Could you check a few things on this model? Use its own coordinates, in mm. A direction names the side the tool comes from. Give positions to 0.01 mm unless a question says otherwise; leave off trailing zeros. Order: outer loops, then holes, each group sorted by start corner. A loop starts at its lowest first (then second) coordinate and runs counter-clockwise, first axis right, second up. Notation, with made-up numbers: M 60.5,10.5 L 99.5,10.5 A23 cw 99.5,28.5 Z; hole C 58,-21.5 d7. An arc over 180 degrees is marked long. Answer in a Markdown table with one row per item. Add a question column.
Autodesk Inventor part; units mm, degrees
ref_plane "Work Plane1" through (0, 0, 8) normal (0, 0, 1) x (1, 0, 0)
ref_plane "YZ Plane" through (0, 0, 0) normal (1, 0, 0) x (0, 1, 0)
ref_plane "XZ Plane" through (0, 0, 0) normal (0, 1, 0) x (-1, 0, 0)
sketch "Sketch1" plane through (0, 0, 0) normal (0, 0, 1) x (1, 0, 0)
  line L0 (-17.75, 0) -> (17.75, 0)
  line L1 (17.75, 0) -> (17.75, -85)
  line L2 (17.75, -85) -> (-17.75, -85)
  line L3 (-17.75, -85) -> (-17.75, 0)
  point P0 (0, 0)
  point P1 (0, 0)
  dimension "d0" = 35.5
  dimension "d1" = 85
extrude "Extrusion1" add sketch "Sketch1" along normal blind 11
sketch "Sketch2" plane through (0, 0, 0) normal (1, 0, 0) x (0, 1, 0)
  line L0 (-85, 0) -> (0, 0)
  line L1 (-85, 0) -> (-85, 11)
  line L2 (0, 11) -> (-85, 11)
  line L3 (0, 0) -> (0, 11)
  line L4 (-85, 82.7102) -> (-37.2472, 0)
  line L5 (0, 0) -> (0, 11)
  line L6 (0, 9) -> (-9, 9)
  line L7 (-9, 9) -> (-13.1212, 7.5)
  line L8 (-13.1212, 7.5) -> (-22, 7.5)
  line L9 (-22, 7.5) -> (-24.7475, 6.5)
  line L10 (-24.7475, 6.5) -> (-41, 6.5)
  line L11 (-45.9075, 15) -> (-85, 15)
  line L12 (-85, 15) -> (-85, 11)
  point P0 (-43.5981, 11)
  dimension "d6" = 60
  dimension "d7" = 20
  dimension "d8" = 2
  dimension "d9" = 3.5
  dimension "d10" = 4.5
  dimension "d11" = 6.5
  dimension "d12" = 9
  dimension "d13" = 13.1212
  dimension "d14" = 24.7475
  dimension "d15" = 22
  dimension "d16" = 41
  dimension "d25" = 15
  dimension "d26" = 4
extrude "Extrusion2" add sketch "Sketch2" along normal mid plane 60 contours L1 L2 L4 L0 | L12 L11 L4 L2
extrude "Extrusion4" add sketch "Sketch2" along normal mid plane 43.6 contours L4 L2 L3 L6 L7 L8 L9 L10
sketch "Sketch3" plane through (0, 0, 0) normal (0, 0, 1) x (1, 0, 0)
  line L0 (-13, 13) -> (13, 13)
  line L1 (-17.75, 0) -> (17.75, 0)
  line L2 (-30, -37.2472) -> (-30, -85)
  line L3 (30, -85) -> (30, -37.2472)
  line L4 (30, -85) -> (-30, -85)
  arc A0 (-13, 13) -> (-30, -4) centre (-13, -4) ccw
  arc A1 (30, -4) -> (13, 13) centre (13, -4) ccw
  line L5 (-30, -37.2472) -> (-30, -4)
  line L6 (30, -37.2472) -> (30, -4)
  point P0 (0, 0)
  dimension "d28" = 13
  dimension "d29" = 17
extrude "Extrusion5" add sketch "Sketch3" against normal blind 3
fillet "Fillet1" radius 3 1 edges at (0, -45.9075, 15)
fillet "Fillet2" radius 2 2 edges at (23.875, -37.2472, 0) (-23.875, -37.2472, 0)
sketch "Sketch4" plane through (0, 0, 11) normal (0, 0, 1) x (1, 0, 0)
  line L0 (21.8, -43.5981) -> (-21.8, -43.5981)
  line L1 (21.8, 0) -> (21.8, -43.5981)
  line L2 (21.8, 0) -> (-21.8, 0)
  line L3 (-21.8, -43.5981) -> (-21.8, 0)
  line L4 (-21.8, -43.5981) -> (-21.8, 0)
  line L5 (-21.8, -9) -> (-17.75, -2)
  line L6 (-21.8, -9) -> (-13.7128, -9) construction
  line L7 (-17.75, -2) -> (-17.75, 0)
  line L8 (21.8, 0) -> (-21.8, 0)
  point P0 (0, 0)
  dimension "d34" = 2
extrude "Extrusion6" cut sketch "Sketch4" against normal up to next contours L3 L2 L7 L5
mirror "Mirror1" about plane through (0, 0, 0) normal (1, 0, 0) of "Extrusion6"
sketch "Sketch5" plane through (0, 0, 11) normal (0, 0, 1) x (1, 0, 0)
  line L0 (0.95, 0) -> (-0.95, 0)
  line L1 (-0.95, 0) -> (-0.95, -17)
  line L2 (-0.95, -17) -> (0.95, -17)
  line L3 (0.95, -17) -> (0.95, 0)
  line L4 (8.45, 0) -> (6.55, 0)
  line L5 (6.55, 0) -> (6.55, -17)
  line L6 (6.55, -17) -> (8.45, -17)
  line L7 (8.45, -17) -> (8.45, 0)
  line L8 (-6.55, 0) -> (-8.45, 0)
  line L9 (-8.45, 0) -> (-8.45, -17)
  line L10 (-8.45, -17) -> (-6.55, -17)
  line L11 (-6.55, -17) -> (-6.55, 0)
  line L12 (17.75, 0) -> (-17.75, 0)
  point P0 (0, 0)
  point P1 (7.5, 0)
  point P2 (-7.5, 0)
  point P3 (0, 0)
  dimension "d37" = 7.5
  dimension "d38" = 7.5
  dimension "d39" = 1.9
  dimension "d40" = 17
extrude "Extrusion7" cut sketch "Sketch5" against normal up to surface (14 mm away)
ref_plane "Work Plane1" through (0, 0, 8) normal (0, 0, 1) x (1, 0, 0)
sketch "Sketch8" plane through (-30, -85, 15) normal (0, 0, 1) x (1, 0, 0)
  line L0 (14.5, 54.9) -> (14.5, 44)
  line L1 (14.5, 44) -> (45.5, 44)
  line L2 (45.5, 44) -> (45.5, 54.9)
  line L3 (45.5, 54.9) -> (42, 54.9)
  line L4 (42, 54.9) -> (42, 49.35)
  line L5 (42, 49.35) -> (18, 49.35)
  line L6 (18, 49.35) -> (18, 54.9)
  line L7 (18, 54.9) -> (14.5, 54.9)
  line L8 (12.5, 4.1) -> (47.5, 4.1)
  line L9 (47.5, 4.1) -> (47.5, 24.6)
  line L10 (47.5, 24.6) -> (12.5, 24.6)
  line L11 (12.5, 24.6) -> (12.5, 4.1)
  arc A0 (12.5, 9.6) -> (18, 4.1) centre (18, 9.6) ccw
  arc A1 (18, 24.6) -> (12.5, 19.1) centre (18, 19.1) ccw
  arc A2 (42, 4.1) -> (47.5, 9.6) centre (42, 9.6) ccw
  arc A3 (47.5, 19.1) -> (42, 24.6) centre (42, 19.1) ccw
  line L12 (12.5, 4.1) -> (12.5, 0)
  line L13 (0, 0) -> (60, 0)
  line L14 (47.5, 4.1) -> (47.5, 0)
  point P0 (30, 85)
  point P1 (30, 44)
  point P2 (30, 24.6)
  dimension "d59" = 41
  dimension "d60" = 31
  dimension "d61" = 5.35
  dimension "d62" = 10.9
  dimension "d63" = 3.5
  dimension "d64" = 19.4
  dimension "d65" = 35
  dimension "d66" = 20.5
  dimension "d67" = 5.5
extrude "Extrusion11" cut sketch "Sketch8" along normal through all both and the other way through all contours L7 L6 L5 L4 L3 L2 L1 L0 | A0 L11 A1 L10 A3 L9 A2 L8
extrude "Extrusion12" cut sketch "Sketch8" against normal blind 5 contours L11 A0 L8 | L8 L14 L13 L12 | A2 L9 L8
sketch "Sketch9" plane through (0, 0, -3) normal (0, 0, -1) x (-1, 0, 0)
  line L0 (15.5, -41) -> (-15.5, -41)
  line L1 (-12, -60.4) -> (12, -60.4)
  arc A0 (17.5, -65.9) -> (12, -60.4) centre (12, -65.9) ccw
  arc A1 (-12, -60.4) -> (-17.5, -65.9) centre (-12, -65.9) ccw
  line L2 (15.5, -41) -> (15.5, -61.6574)
  line L3 (30, -37.8246) -> (17.75, -37.8246)
  line L4 (-15.5, -41) -> (-15.5, -61.6574)
  point P0 (0, 0)
extrude "Extrusion13" cut sketch "Sketch9" against normal blind 11.5
equation "\"overprint\" = 0.1"
properties part number "gehaeuse"
1. If I drill on line 1 along X through (y, z) = (-7, 3.25); line 2 along Y through (x, z) = (5.5, 9.75); line 3 along Y through (x, z) = (-9.5, 1.5), over which ranges is the centre line in solid material (lowest first)? Write a range as [from, to].
2. Suppose I cut it at B-B on x = -11. List the corners of the cut face in (y, z) for me.
3. Thinking about a two-plate mould opening in Z: for faces 4 (the flat face through (-20, -33, 6.5)), 5 (the flat face through (-8.45, -8, 4)), 6 (the cylindrical face through (-0.42, -46.16, 14.61)), which applies, pulls with the +Z half, pulls with the -Z half, needs draft (parallel to the pull), parting line crosses it, or undercut?
4. Will these pins go through, and if not, where does the flat tip stop? P1, Ø5, axis at x = 2, y = -40.5, coming from the +Z side; P2, Ø10, axis at y = -4.5, z = 12.5, coming from the +X side; P3, Ø4, axis at x = 17.5, z = 0, coming from the +Y side.
5. Suppose I cut it at A-A on y = -32. List the corners of the cut face in (x, z) for me, plus the area to 3 significant figures.
6. Suppose I cut it at C-C on y = -8. List the corners of the cut face in (x, z) for me.
7. For faces 1 (the flat face through (0, -82, 10)), 2 (the flat face through (19.75, -11.03, 8.26)), 3 (the flat face through (6.55, -8, 4)), which set-ups out of +Z, -Z, +X, -X, +Y, -Y let a thin tool reach every point of the face, with its end or its side?
Findings below:
| question | item | result |
|---|---|---|
| 1 | line 1 | [-17.75, -8.45], [-6.55, -0.95], [0.95, 6.55], [8.45, 17.75] |
| 1 | line 2 | [-85, -80.9], [-60.4, -41], [-35.65, 0] |
| 1 | line 3 | [-85, -80.9], [-35.65, 0] |
| 2 | outline | M -85,-3 L -80.9,-3 L -80.9,10 L -85,10 Z; M -60.4,8.5 L -41,8.5 L -41,11 L -43.6,11 L -45.04,13.5 A3 ccw -47.64,15 L -60.4,15 Z; M -35.65,-3 L 13,-3 L 13,0 L 0,0 L 0,11 L -35.65,11 Z |
| 3 | face 4 | undercut |
| 3 | face 5 | needs draft |
| 3 | face 6 | pulls with the +Z half |
| 4 | P1 | z = 11 |
| 4 | P2 | x = 21.8 |
| 4 | P3 | y = 12.82 |
| 5 | outline | M -30,-3 L -15.5,-3 L -15.5,11 L -21.8,11 L -21.8,6.5 L -17.75,6.5 L -17.75,0 L -30,0 Z; M -12,-3 L 12,-3 L 12,11 L -12,11 Z; M 15.5,-3 L 30,-3 L 30,0 L 17.75,0 L 17.75,6.5 L 21.8,6.5 L 21.8,11 L 15.5,11 Z |
| 5 | area | 509 mm2 |
| 6 | outline | M -30,-3 L -8.45,-3 L -8.45,11 L -21.22,11 L -21.22,9 L -17.75,9 L -17.75,0 L -30,0 Z; M -6.55,-3 L -0.95,-3 L -0.95,11 L -6.55,11 Z; M 0.95,-3 L 6.55,-3 L 6.55,11 L 0.95,11 Z; M 8.45,-3 L 30,-3 L 30,0 L 17.75,0 L 17.75,9 L 21.22,9 L 21.22,11 L 8.45,11 Z |
| 7 | face 1 | +Z, -Y |
| 7 | face 2 | +X, +Y |
| 7 | face 3 | +Z, -Z |
